```python
from build123d import *

# Parameters (mm, degrees)
SKETCH_1_R      = 10.9
SKETCH_1_R_2    = 9.4
EXTRUDE_1_DEPTH = 2.5
SKETCH_3_R      = 1.25
FILLET_1_R      = 1


with BuildPart() as part:
    # 草图1 → 凸台-拉伸1 (new body, symmetric)
    with BuildSketch(Plane.XY):
        Circle(SKETCH_1_R)
        Circle(SKETCH_1_R_2, mode=Mode.SUBTRACT)
    extrude(amount=EXTRUDE_1_DEPTH, both=True)

    # 草图3 → 切除-旋转1 (revolve, cut)
    with BuildSketch(Plane(origin=(0, 0, 0), x_dir=(1, 0, 0), z_dir=(0, 1, 0))):
        with Locations((-8.9, 0)):
            Circle(SKETCH_3_R)
    revolve(axis=Axis((0, 0, 2.5), (0, 0, -1)), mode=Mode.SUBTRACT)

    # 圆角1
    fillet_1_edges = [part.edges().sort_by_distance(p)[0] for p in [
        (0, 9.4, 1.145643924),
        (0, -9.4, -1.145643924),
    ]]
    fillet(fillet_1_edges, radius=FILLET_1_R)


solid = part.part
```
The listing builds one solid part. Answer for the finished solid, in the listing's coordinates (mm). Coordinates: 2 decimals unless noted, no trailing zeros. Return JSON: item names as keys, results as strings. Group by question number.
1. Determine the mould class of faces 1 (the flat face through (-10, 0, -2.5)), 2 (the cylindrical face through (-7.46, -5.72, 2.08)), 3 (the cylindrical face through (10.4, 3.27, 0.04)) for opening direction Y: released by +Y, released by -Y, zero draft, split by the parting line, or undercut.
2. Straight lines are drawn through the part: L1, parallel to Y at x = 0, z = -2.2; L2, parallel to Y at x = -3.5, z = 1.5; L3, parallel to X at y = 5, z = -1.7. For each, find the intervals that lie inside material, in ascending order.
3. Given pin 1 (1.5 mm diameter, centred on y = -1.5, z = -0.5, fed in from +X); pin 2 (3 mm diameter, centred on y = -1, z = -1.5, fed in from -X); pin 3 (2 mm diameter, centred on x = -4.5, z = -1.5, fed in from +Y), each flat-ended and moving along its own axis, determine where each tip first touches the part or whether it passes through.
Ans:
{
 "1": {"face 1": "zero draft", "face 2": "undercut", "face 3": "split by the parting line"},
 "2": {"L1": "-10.9 to -9.4, 9.4 to 10.9", "L2": "-10.32 to -8.74, 8.74 to 10.32", "L3": "-9.69 to -7.96, 7.96 to 9.69"},
 "3": {"pin 1": "x = 10.87", "pin 2": "x = -10.9", "pin 3": "y = 10.32"}
}
